Can you work these out from the model? Positions are in its coordinate system, mm. Face numbers are marked on the shaded views. Round coordinates to 2 decimals unless told otherwise and drop trailing zeros. Order: outer loops, then holes, each group sorted by start corner. A loop starts at its lowest first (then second) coordinate and runs counter-clockwise, first axis right, second up. Notation, with made-up numbers: M 11.5,45.25 L 49.5,45.25 A20 ccw 49.5,71.25 Z; hole C -14.75,89 d11. An arc over 180 degrees is marked long. Answer as a JSON object with one key per item and string values. Group by question number.
from build123d import *

# Parameters (mm, degrees)
F0_W          = 76
F0_H          = 144
F1_DEPTH      = 13
F3_DEPTH      = 142
F4_W          = 64
F4_H          = 2
F5_DEPTH      = 4
F6_W          = 10.5
F6_H          = 7.5
F7_DEPTH      = 25
F8_W          = 8.0420786627
F8_H          = 42
F9_DEPTH      = 25
F11_DEPTH     = 76
F12_T4_DEPTH  = 76
F12_T10_DEPTH = 76
F12_T16_DEPTH = 76
F12_T23_DEPTH = 76
F12_T29_DEPTH = 76


# Not quite as in the source:
# - a fillet or chamfer that OpenCascade refuses, or shapes differently, is made with other operations: its cross-section is extruded or revolved along the edge and cut away or added


with BuildPart() as f1:
    # F0 (on Front) → F1 (new body)
    with BuildSketch(Plane.XZ):
        Rectangle(F0_W, F0_H)
    extrude(amount=F1_DEPTH)

    # F2 (on face) → F3 (cut)
    with BuildSketch(Plane.XY.offset(72)):
        Polygon((-32, -11), (-32, -13), (32, -13), (32, -11), (36, -11), (36, -2), (-36, -2), (-36, -11), align=None)
    extrude(amount=-F3_DEPTH, mode=Mode.SUBTRACT)

    # F4 (on face) → F5 (join)
    with BuildSketch(Plane.XY.offset(-70)):
        with Locations((0, -12)):
            Rectangle(F4_W, F4_H)
    extrude(amount=F5_DEPTH)

    # F6 (on face) → F7 (cut)
    with BuildSketch(Plane(origin=(0, 0, -72), x_dir=(1, 0, 0), z_dir=(0, 0, -1))):
        with Locations((0, 6.5)):
            Rectangle(F6_W, F6_H)
    extrude(amount=-F7_DEPTH, mode=Mode.SUBTRACT)

    # F8 (on face) → F9 (cut)
    with BuildSketch(Plane.YZ.offset(38)):
        with Locations((-6.5, 20)):
            Rectangle(F8_W, F8_H)
    extrude(amount=-F9_DEPTH, mode=Mode.SUBTRACT)

    # F10 (on face) → F11 (join)
    with BuildSketch(Plane.YZ.offset(38)):
        Polygon((-33.1302755044, -68.4504892995), (-13, -72), (-13, -69.4614334703), (-32.6961550602, -65.9884699169), align=None)
    extrude(amount=-F11_DEPTH)

    # F12: chamfer of 5 on 1 edges, made by hand


with BuildPart() as f12_tool2:
    # F12_s3 → F12_t4 (new body)
    with BuildSketch(Plane.YZ.offset(38)):
        Polygon((-13, -64.4614334703), (-17.9240387651, -68.593192582), (-13, -69.4614334703), align=None)
    extrude(amount=-F12_T4_DEPTH)

    split(bisect_by=Plane.XY.offset(-66), keep=Keep.TOP)

    split(bisect_by=Plane.YZ.offset(32), keep=Keep.TOP)


with BuildPart() as f1_1:
    add(f1.part)

    # F12_t1: union F12_tool2
    add(f12_tool2.part)


with BuildPart() as f12_tool8:
    # F12_s9 → F12_t10 (new body)
    with BuildSketch(Plane.YZ.offset(38)):
        Polygon((-13, -64.4614334703), (-17.9240387651, -68.593192582), (-13, -69.4614334703), align=None)
    extrude(amount=-F12_T10_DEPTH)

    split(bisect_by=Plane.XY.offset(-66), keep=Keep.BOTTOM)

    split(bisect_by=Plane.YZ.offset(32), keep=Keep.TOP)


with BuildPart() as f1_2:
    add(f1_1.part)

    # F12_t7: union F12_tool8
    add(f12_tool8.part)


with BuildPart() as f12_tool14:
    # F12_s15 → F12_t16 (new body)
    with BuildSketch(Plane.YZ.offset(38)):
        Polygon((-13, -64.4614334703), (-17.9240387651, -68.593192582), (-13, -69.4614334703), align=None)
    extrude(amount=-F12_T16_DEPTH)

    split(bisect_by=Plane.YZ.offset(-32), keep=Keep.TOP)

    split(bisect_by=Plane.XY.offset(-66), keep=Keep.BOTTOM)

    split(bisect_by=Plane.YZ.offset(32), keep=Keep.BOTTOM)


with BuildPart() as f1_3:
    add(f1_2.part)

    # F12_t13: union F12_tool14
    add(f12_tool14.part)


with BuildPart() as f12_tool21:
    # F12_s22 → F12_t23 (new body)
    with BuildSketch(Plane.YZ.offset(38)):
        Polygon((-13, -64.4614334703), (-17.9240387651, -68.593192582), (-13, -69.4614334703), align=None)
    extrude(amount=-F12_T23_DEPTH)

    split(bisect_by=Plane.YZ.offset(-32), keep=Keep.BOTTOM)

    split(bisect_by=Plane.XY.offset(-66), keep=Keep.TOP)


with BuildPart() as f1_4:
    add(f1_3.part)

    # F12_t20: union F12_tool21
    add(f12_tool21.part)


with BuildPart() as f12_tool27:
    # F12_s28 → F12_t29 (new body)
    with BuildSketch(Plane.YZ.offset(38)):
        Polygon((-13, -64.4614334703), (-17.9240387651, -68.593192582), (-13, -69.4614334703), align=None)
    extrude(amount=-F12_T29_DEPTH)

    split(bisect_by=Plane.YZ.offset(-32), keep=Keep.BOTTOM)

    split(bisect_by=Plane.XY.offset(-66), keep=Keep.BOTTOM)


with BuildPart() as f1_5:
    add(f1_4.part)

    # F12_t26: union F12_tool27
    add(f12_tool27.part)


solid = f1_5.part
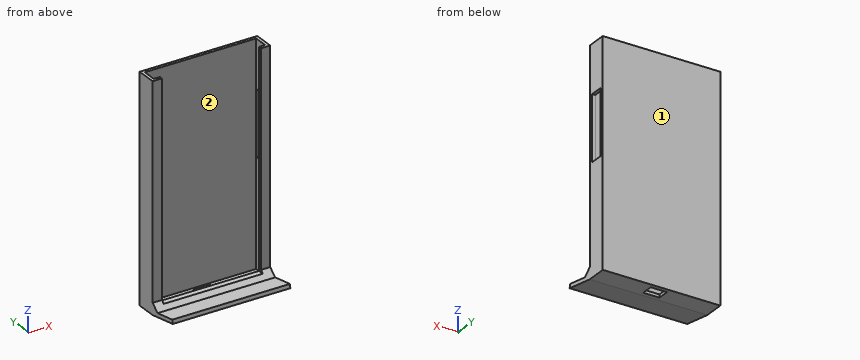
Item 1: Suppose I cut it at B-B, the plane x = -22. Write out the boundary of the cut face in (y, z).
Item 2: Suppose I cut it at A-A, the plane z = 10.5. Write out the boundary of the cut face in (x, y).
Item 3: If we mould it in two halves opening along X, with no side actions, what happens to the marked faces 1 and 2? For each: +X half, -X half, draft (parallel to the pull), parting line (faces both ways), or undercut.
Item 4: Suppose I cut it at D-D, the plane y = -27.5. Write out the boundary of the cut face in (x, z), and give its area (3 significant figures).
Item 5: I need wall thicknesses on line 1 (X direction, y = -4.5, z = 60); line 2 (Y direction, x = -21, z = 7); line 3 (Z direction, x = 20, y = -10). Which ranges of each line are inside material? Lowest first, please.
Item 6: Suppose I cut it at C-C, the plane z = -61. Write out the boundary of the cut face in (x, y), and give its area (3 significant figures).
Item 7: I'm going to push flat-ended pins straight in: pin 1 Ø3 at (x, z) = (36, 11.5) entering from -Y; pin 2 Ø1 at (x, y) = (-2, -22) entering from +Z; pin 3 Ø4.5 at (x, y) = (-6, -7.5) entering from +Z. Where does each tip first touch, or does it pass through?
Computed:
{
 "1": {"outline": "M -33.13,-68.45 L -13,-72 L 0,-72 L 0,72 L -2,72 L -2,-70 L -11,-70 L -11,-66 L -14.83,-66 L -17.92,-68.59 L -32.7,-65.99 Z"},
 "2": {"outline": "M -38,-13 L -32,-13 L -32,-11 L -36,-11 L -36,-2 L 36,-2 L 36,-2.48 L 38,-2.48 L 38,0 L -38,0 Z; M 32,-13 L 38,-13 L 38,-10.52 L 36,-10.52 L 36,-11 L 32,-11 Z"},
 "3": {"face 1": "draft", "face 2": "undercut"},
 "4": {"outline": "M -38,-69.44 L 38,-69.44 L 38,-66.9 L -38,-66.9 Z", "area": "193 mm^2"},
 "5": {"line 1": "x = -38 to -36, 36 to 38", "line 2": "y = -2 to 0", "line 3": "z = -72 to -70"},
 "6": {"outline": "M -38,-13 L -32,-13 L -32,-11 L -36,-11 L -36,-2 L 36,-2 L 36,-11 L 32,-11 L 32,-13 L 38,-13 L 38,0 L -38,0 Z", "area": "212 mm^2"},
 "7": {"pin 1": "stops at y = -13", "pin 2": "stops at z = -67.79", "pin 3": "stops at z = -70"}
}
